Design review of the part built by this model. Coordinates are the model's own, in mm. Face numbers are marked on the shaded views. Give positions to 0.01 mm unless a question says otherwise; leave off trailing zeros. Order: outer loops, then holes, each group sorted by start corner. A loop starts at its lowest first (then second) coordinate and runs counter-clockwise, first axis right, second up. Notation, with made-up numbers: (5.5, 60) -> (20.5, 60) arc R27 cw to (20.5, 93) -> close; hole circle Ø11 at (65.25, 26). An arc over 180 degrees is marked (long way). One line per item, written item: value. Start each with the question number.
1) Consider section D-D (z = 15). State the section outline as (x, y) points, plus the area to 3 significant figures.
2) Wall thickness on line 1 along X through (y, z) = (0, 1.9); line 2 along Y through (x, z) = (4.5, 3): over which ranges is each line inside the solid? List them lowest first. Write a range as from..to.
3) The part is to be moulded in two halves that separate along Y. For the marked faces 1, 2, 3 and 4, say which applies: released by +Y, released by -Y, zero draft, split by the parting line, or undercut.
4) For pin 1 (3 mm diameter, centred on x = 7, z = 17, fed in from +Y); pin 2 (5 mm diameter, centred on x = -7.5, z = 7.5, fed in from +Y); pin 3 (12 mm diameter, centred on x = 3.5, y = -9.5, fed in from +Z), all flat-tipped, find the tip position at first contact; note any pin that passes through.
5) Consider section A-A (y = 0). State the section outline as (x, z) points.
6) Consider section C-C (z = 25.5). State the section outline as (x, y) points.
from build123d import *

# Parameters (mm, degrees)
F2_R     = 4
F3_DEPTH = 3
F4_R     = 4
F5_DEPTH = 3


with BuildPart() as f1:
    # F0 (on Front) → F1 (revolve)
    with BuildSketch(Plane.XZ):
        Polygon((0, 25), (0, 0), (12.5, 0), (12.5, 5), (4, 25), align=None)
    revolve(axis=Axis((0, 0, 12.5), (0, 0, -1)))

    # F2 (on face) → F3 (join)
    with BuildSketch(Plane.XY.offset(25)):
        Circle(F2_R)
    extrude(amount=F3_DEPTH)

    # F4 (on face) → F5 (cut)
    with BuildSketch(Plane(origin=(0, 0, 0), x_dir=(1, 0, 0), z_dir=(0, 0, -1))):
        Circle(F4_R)
    extrude(amount=-F5_DEPTH, mode=Mode.SUBTRACT)


solid = f1.part
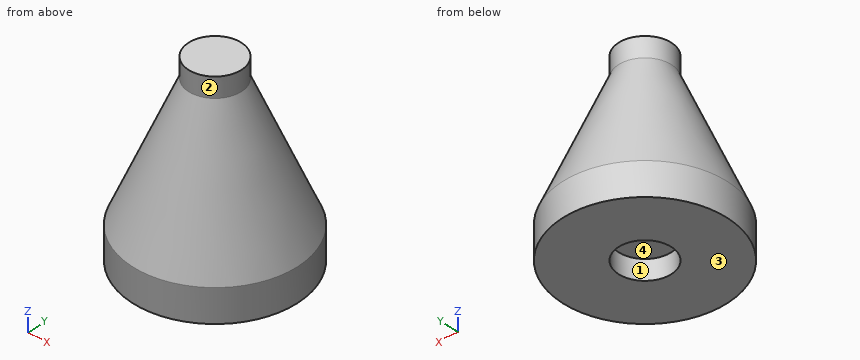
Checked values:
1. outline: circle Ø16.5 at (0, 0)
1. area: 214 mm^2
2. line 1: x = -12.5..-4, 4..12.5
2. line 2: y = -11.66..11.66
3. face 1: undercut
3. face 2: split by the parting line
3. face 3: zero draft
3. face 4: undercut
4. pin 1: stops at y = 5.2
4. pin 2: stops at y = 10.76
4. pin 3: stops at z = 24.71
5. outline: (-12.5, 0) -> (-4, 0) -> (-4, 3) -> (4, 3) -> (4, 0) -> (12.5, 0) -> (12.5, 5) -> (4, 25) -> (4, 28) -> (-4, 28) -> (-4, 25) -> (-12.5, 5) -> close
6. outline: circle Ø8 at (0, 0)
